```python
from build123d import *

# Parameters (mm, degrees)
BOSS_EXTRUDE1_DEPTH            = 4
DRAFT1_ANGLE                   = 45.000000004
DRAFT2_ANGLE                   = 45.000000005
F_4_1_4_1_DIAMETER_HOLE1_D     = 4.1
F_4_1_4_1_DIAMETER_HOLE1_DEPTH = 4
F_2_7_2_7_DIAMETER_HOLE1_D     = 2.7
F_2_7_2_7_DIAMETER_HOLE1_DEPTH = 4
FILLET1_R                      = 1
FILLET2_R                      = 6.5


with BuildPart() as part:
    # Sketch1 → Boss-Extrude1 (new body)
    with BuildSketch(Plane.XZ.offset(2)):
        with BuildLine():
            Line((11.124319466, 26.5), (-6.5, 26.5))
            Line((-6.5, 26.5), (-6.5, 0))
            ThreePointArc((-6.5, 0), (3e-09, -6.500000003), (6.500000005, 0))
            Line((6.500000005, 0), (6.500000005, 20.5))
            Line((6.500000005, 20.5), (13.60960084, 20.5))
            Line((13.60960084, 20.5), (13.60960084, 36.100603473))
            Line((13.60960084, 36.100603473), (11.124319466, 38.585884847))
            Line((11.124319466, 38.585884847), (11.124319466, 26.5))
        make_face()
    extrude(amount=-BOSS_EXTRUDE1_DEPTH)

    # Draft1
    draft1_faces = [part.faces().sort_by_distance(p)[0] for p in [
        (13.60960084, 0, 28.300301737),
    ]]
    draft(draft1_faces, Plane(origin=(6.500000005, 2, 20.5), x_dir=(-1, 0, 0), z_dir=(0, 0, -1)), DRAFT1_ANGLE)

    # Draft2
    draft2_faces = [part.faces().sort_by_distance(p)[0] for p in [
        (11.124319466, 0, 32.542942424),
    ]]
    draft(draft2_faces, Plane(origin=(11.124319466, 2, 26.5), x_dir=(1, 0, 0), z_dir=(0, 0, 1)), DRAFT2_ANGLE)

    # Sketch2 → Cut-Revolve1 (revolve, cut)
    with BuildSketch(Plane.XY.offset(20)):
        Polygon((6, 2), (0, 2), (0, -2), (6, -2), (6, -1), (5, -1), (5, 1), (6, 1), align=None)
    revolve(axis=Axis((0, 2, 20), (0, -1, 0)), mode=Mode.SUBTRACT)

    # Ø4.1 (4.1) Diameter Hole1
    with Locations(Plane(origin=(0, 2, 0), x_dir=(1, 0, 0), z_dir=(0, 1, 0))):
        with Locations((0, 2.5)):
            Hole(F_4_1_4_1_DIAMETER_HOLE1_D / 2, depth=F_4_1_4_1_DIAMETER_HOLE1_DEPTH)

    # Ø2.7 (2.7) Diameter Hole1
    with Locations(Plane(origin=(0, -2, 0), x_dir=(-1, 0, 0), z_dir=(0, -1, 0))):
        with Locations((-14.692388155, -24.41121444), (-18.227922061, -27.946748346)):
            Hole(F_2_7_2_7_DIAMETER_HOLE1_D / 2, depth=F_2_7_2_7_DIAMETER_HOLE1_DEPTH)

    # Fillet1
    fillet1_edges = [part.edges().sort_by_distance(p)[0] for p in [
        (13.60960084, 0, 20.5),
        (6.500000005, 0, 20.5),
        (11.124319466, 0, 26.5),
    ]]
    fillet(fillet1_edges, radius=FILLET1_R)

    # Fillet2
    fillet2_edges = [part.edges().sort_by_distance(p)[0] for p in [
        (-6.5, 0, 26.5),
    ]]
    fillet(fillet2_edges, radius=FILLET2_R)


solid = part.part
```
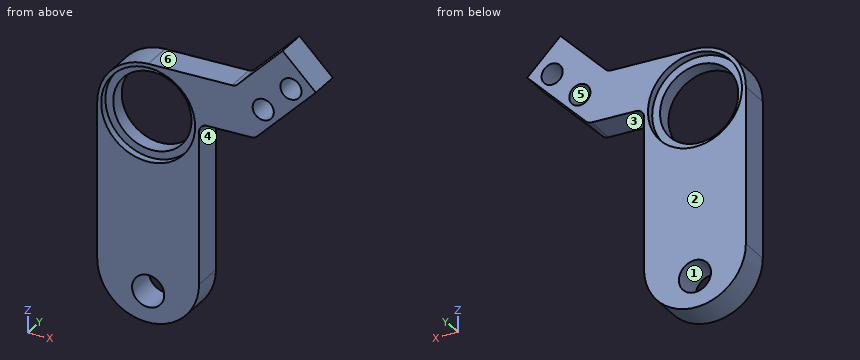
The model under review builds one solid part; all positions refer to its coordinate system, in mm. Face numbers are marked on the shaded views. A direction names the side the tool comes from. Round coordinates to 2 decimals unless told otherwise and drop trailing zeros. Order: outer loops, then holes, each group sorted by start corner. A loop starts at its lowest first (then second) coordinate and runs counter-clockwise, first axis right, second up.
Item 1: Add section D-D, the plane x = 3.75. State the section outline as (y, z) points.
Working result:
outline: (-2, -5.31) - (2, -5.31) - (2, 15.32) - (1, 15.32) - (1, 16.69) - (-1, 16.69) - (-1, 15.32) - (-2, 15.32) - close; (-2, 24.68) - (-1, 24.68) - (-1, 23.31) - (1, 23.31) - (1, 24.68) - (2, 24.68) - (2, 26.5) - (-2, 26.5) - close
Item 2: For pin 1 (14 mm diameter, centred on x = 0, z = 20, fed in from -Y); pin 2 (1.5 mm diameter, centred on x = 11, y = 0.5, fed in from +Z); pin 3 (12 mm diameter, centred on x = 15.5, z = 2.5, fed in from -Y); pin 4 (11 mm diameter, centred on x = 0, z = 20, fed in from -Y), all flat-tipped, find the tip position at first contact; note any pin that passes through.
Working result:
pin 1: stops at y = -2
pin 2: stops at z = 27.13
pin 3: passes through
pin 4: stops at y = -1
Item 3: Add section C-C, the plane y = -0.05. State the section outline as (x, z) points.
Working result:
outline: (-6.5, 0) arc R6.5 ccw to (6.5, 0) - (6.5, 19.5) arc R1 cw to (7.5, 20.5) - (13.2, 20.5) arc R1 ccw to (13.9, 20.79) - (21.41, 28.3) - (17.17, 32.54) - (11.42, 26.79) arc R1 cw to (10.71, 26.5) - (0, 26.5) arc R6.5 ccw to (-6.5, 20) - close; hole circle Ø10 at (0, 20); hole circle Ø4.1 at (0, -2.5); hole circle Ø2.7 at (14.69, 24.41); hole circle Ø2.7 at (18.23, 27.95)
Item 4: Add section A-A, the plane z = -2.5. State the section outline as (x, y) points, and give its area (3 significant figures).
Working result:
outline: (-6, -2) - (-2.05, -2) - (-2.05, 2) - (-6, 2) - close; (2.05, -2) - (6, -2) - (6, 2) - (2.05, 2) - close
area: 31.6 mm2
Item 5: To check wall thickness, follow probe 1 along Z at (x, y) = (0, 1.45); probe 2 along Z at (x, y) = (0, 0.5); probe 3 along Z at (x, y) = (10.75, 0.9). State the ranges of each line that lie inside material, in increasing order.
Working result:
probe 1: z = -6.5 to -4.55, -0.45 to 14, 26 to 26.5
probe 2: z = -6.5 to -4.55, -0.45 to 15, 25 to 26.5
probe 3: z = 20.5 to 26.5
Item 6: Add section B-B, the plane x = -4.5. State the section outline as (y, z) points, and give its area (3 significant figures).
Working result:
outline: (-2, -4.69) - (2, -4.69) - (2, 16.03) - (1, 16.03) - (1, 17.82) - (-1, 17.82) - (-1, 16.03) - (-2, 16.03) - close; (-2, 23.97) - (-1, 23.97) - (-1, 22.18) - (1, 22.18) - (1, 23.97) - (2, 23.97) - (2, 24.69) - (-2, 24.69) - close
area: 92.9 mm2
Item 7: Draft analysis for pull direction Z (two halves, no side actions). For the marked faces 1, 2 and 3, state which applies: released by +Z, released by -Z, zero draft, split by the parting line, or undercut.
Working result:
face 1: undercut
face 2: zero draft
face 3: released by -Z
Item 8: Machinability: for the marked faces 4, 5 and 6, which of the approach directions +Z, -Z, +X, -X, +Y, -Y give a long, thin tool a straight path to every point of the face, cutting with its end or side? Answer none if there is none.
Working result:
face 4: -Z, +X, +Y, -Y
face 5: +Y, -Y
face 6: +Z, -X, +Y, -Y
